The model under review builds one solid part; all positions refer to its coordinate system, in mm. A direction names the side the tool comes from. Round coordinates to 2 decimals unless told otherwise and drop trailing zeros. Write each loop counter-clockwise with the first axis right and the second up, starting at its lowest first coordinate (ties: lowest second). Pieces come first, ordered by that corner, then holes. Notation, with made-up numbers: M -38.75,-20 L -2.75,-20 A28 cw -2.75,19 Z; hole C -10.5,-16.5 d2. An arc over 180 degrees is marked long. One line per item, written item: value. Start each with the question number.
1) Wall thickness on probe 1 along Z at (x, y) = (176.5, 3); probe 2 along Z at (x, y) = (95, 1.5); probe 3 along X at (y, z) = (3, 41): over which ranges is each line inside the solid? List them lowest first.
2) Tool access review of faces 1 (the face through (215.9, 3, 25)), 2 (the face through (9.323, 3.219, 12.774)), 3 (the face through (165.1, 3, 38)): name each direction out of +Z, -Z, +X, -X, +Y, -Y from which nothing blocks a thin tool from reaching the whole face with its end or side.
3) Mouldability with a two-part tool opening along Z and no side actions: class faces 4 (the face through (100, 3, 16.078)), 5 (the face through (187.527, 3.219, 12.626)), 6 (the face through (133, 0, 19)), 7 (the face through (191, 3, 50.8)) as +Z half, -Z half, draft (parallel to the pull), parting line (faces both ways), or undercut.
4) Take a section at D-D, the plane z = 28. Write out the cut boundary in (x, y), and give its area (3 significant figures).
5) For P1, Ø1.9, axis at y = 2.5, z = 40.5, coming from the -X side; P2, Ø4, axis at x = 207.96, z = 34.92, coming from the -Y side, all flat-tipped, find the tip position at first contact; note any pin that passes through.
6) Take a section at B-B, the plane x = 29.5. Write out the cut boundary in (y, z).
7) Take a section at A-A, the plane z = 12.7. Write out the cut boundary in (x, y), and give its area (3 significant figures).
8) Take a section at C-C, the plane y = 5. State how many separate pieces and enclosed holes the cut face has, and give its area (3 significant figures).
from build123d import *

# Parameters (mm, degrees)
BOSS_EXTRUDE1_DEPTH                            = 6.35
CUT_EXTRUDE1_DEPTH                             = 222.886846163
CSK_FOR_4_FLAT_HEAD_MACHINE_SCREW1_D           = 3.2639
CSK_FOR_4_FLAT_HEAD_MACHINE_SCREW1_CSINK_D     = 5.715
CSK_FOR_4_FLAT_HEAD_MACHINE_SCREW1_CSINK_ANGLE = 82


with BuildPart() as part:
    # Sketch1 → Boss-Extrude1 (new body)
    with BuildSketch(Plane(origin=(0, 0, 0), x_dir=(1, 0, 0), z_dir=(0, 1, 0))):
        Polygon((0, 0), (215.9, 0), (215.9, -50.8), (165.1, -50.8), (165.1, -25.4), (0, -25.4), align=None)
    extrude(amount=BOSS_EXTRUDE1_DEPTH)

    # Sketch2 → Cut-Extrude1 (cut, through all)
    with BuildSketch(Plane(origin=(0, 6.35, 0), x_dir=(1, 0, 0), z_dir=(0, 1, 0))):
        with BuildLine():
            Line((184.15, -16.0782), (12.7, -16.0782))
            ThreePointArc((12.7, -16.0782), (9.3218, -12.7), (12.7, -9.3218))
            Line((12.7, -9.3218), (184.15, -9.3218))
            ThreePointArc((184.15, -9.3218), (187.5282, -12.7), (184.15, -16.0782))
        make_face()
    extrude(amount=-CUT_EXTRUDE1_DEPTH, mode=Mode.SUBTRACT)

    # CSK for #4 Flat Head Machine Screw1 (through all)
    with Locations(Plane(origin=(0, 0, 0), x_dir=(-1, 0, 0), z_dir=(0, -1, 0))):
        with Locations((-207.9625, -34.925), (-207.9625, -41.275)):
            CounterSinkHole(CSK_FOR_4_FLAT_HEAD_MACHINE_SCREW1_D / 2, CSK_FOR_4_FLAT_HEAD_MACHINE_SCREW1_CSINK_D / 2, counter_sink_angle=CSK_FOR_4_FLAT_HEAD_MACHINE_SCREW1_CSINK_ANGLE)


solid = part.part
Checked values:
1. probe 1: z = 0 to 9.32, 16.08 to 50.8
1. probe 2: z = 0 to 9.32, 16.08 to 25.4
1. probe 3: x = 165.1 to 206.35, 209.57 to 215.9
2. face 1: +Z, -Z, +X, +Y, -Y
2. face 2: +Y, -Y
2. face 3: +Z, -X, +Y, -Y
3. face 4: undercut
3. face 5: undercut
3. face 6: draft
3. face 7: +Z half
4. outline: M 165.1,0 L 215.9,0 L 215.9,6.35 L 165.1,6.35 Z
4. area: 323 mm2
5. P1: stops at x = 165.1
5. P2: stops at y = 0.98
6. outline: M 0,0 L 6.35,0 L 6.35,9.32 L 0,9.32 Z; M 0,16.08 L 6.35,16.08 L 6.35,25.4 L 0,25.4 Z
7. outline: M 0,0 L 9.32,0 L 9.32,6.35 L 0,6.35 Z; M 187.53,0 L 215.9,0 L 215.9,6.35 L 187.53,6.35 Z
7. area: 239 mm2
8. separate pieces: 1
8. enclosed holes: 3
8. area: 5,560 mm2
